from build123d import *

# Parameters (mm, degrees)
BASEHEAD_DEPTH = 13.4
SKETCH4_W      = 0.8
SKETCH4_H      = 12.320508076


# Read off the part's stored shape, not the designer's step: HeadChamfer
with BuildPart() as part:
    # Sketch1 → BaseHead (new body)
    with BuildSketch(Plane(origin=(0, 0, 0), x_dir=(0, 0, -1), z_dir=(1, 0, 0))):
        Polygon((15, 8.660254038), (15, -8.660254038), (0, -17.320508076), (-15, -8.660254038), (-15, 8.660254038), (0, 17.320508076), align=None)
    extrude(amount=BASEHEAD_DEPTH)

    # HeadChamfer outline → HeadChamfer (revolve, cut)
    with BuildSketch(Plane.YX):
        Polygon((17.320508077, 1.339745963), (14.99999979, -1.21e-07), (17.320508077, -1.21e-07), align=None)
    revolve(axis=Axis((0, 0, 0), (1, 0, 0)), mode=Mode.SUBTRACT)

    # HeadChamfer 2 outline → HeadChamfer 2 (revolve)
    with BuildSketch(Plane.YX):
        Polygon((10, 13.4), (10, 172.026), (8.626, 173.4), (0, 173.4), (0, 13.4), align=None)
    revolve(axis=Axis((0, 0, 0), (1, 0, 0)))

    # Sketch4 → BearingFace (revolve, cut)
    with BuildSketch(Plane.XY, mode=Mode.PRIVATE) as bearingface_sk:
        with Locations((13, 21.160254038)):
            Rectangle(SKETCH4_W, SKETCH4_H)
    revolve(bearingface_sk.sketch.rotate(Axis((0, 0, 0), (1, 0, 0)), 90), axis=Axis((0, 0, 0), (1, 0, 0)), mode=Mode.SUBTRACT)


solid = part.part
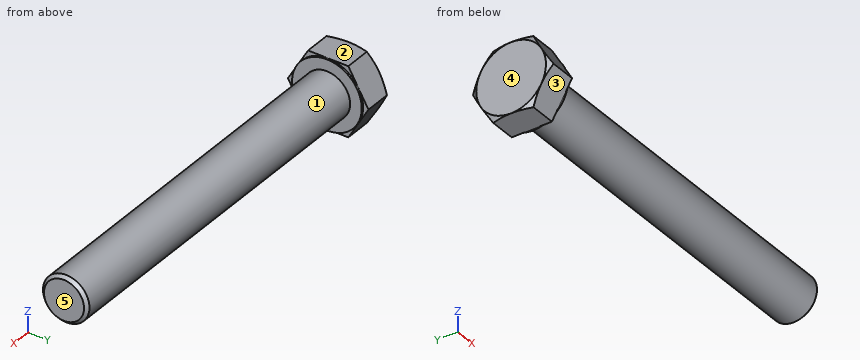
Could you check a few things on this model? Use its own coordinates, in mm. Face numbers are marked on the shaded views. A direction names the side the tool comes from. Give positions to 0.01 mm unless a question says otherwise; leave off trailing zeros. Order: outer loops, then holes, each group sorted by start corner. A loop starts at its lowest first (then second) coordinate and runs counter-clockwise, first axis right, second up. Notation, with made-up numbers: (71, 52) - (78, 52) arc R29 ccw to (78, 77) - close; hole circle Ø10 at (84.25, 26). An arc over 180 degrees is marked (long way). One line per item, written item: value. Start each with the question number.
1. If I drill on probe 1 along X at (y, z) = (10, -5); probe 2 along Z at (x, y) = (89.5, 0); probe 3 along Y at (x, z) = (144.5, 5.5), over which ranges is the centre line in solid material (lowest first)?
2. For the marked faces 1 and 2, which set-ups out of +Z, -Z, +X, -X, +Y, -Y let a thin tool reach every point of the face, with its end or its side?
3. Imagine slicing it at A-A on x = 127. List the corners of the cut face in (y, z) for me, plus the area to 3 significant figures.
4. Thinking about a two-plate mould opening in X: for the marked faces 3, 4 and 5, which applies, +X half, -X half, draft (parallel to the pull), parting line (faces both ways), or undercut?
5. For P1, Ø8, axis at x = 102, y = -2.5, coming from the +Z side; P2, Ø2, axis at y = -4, z = 9.5, coming from the +X side; P3, Ø5, axis at x = 113.5, z = 11, coming from the -Y side, each with a flat end and sliding along its axis, tell me the tip position at first contact or that it passes through.
Values:
1. probe 1: 0 to 13.4
1. probe 2: -10 to 10
1. probe 3: -8.35 to 8.35
2. face 1: +X
2. face 2: +Z, +X, -X, +Y, -Y
3. outline: circle Ø20 at (0, 0)
3. area: 314 mm²
4. face 3: draft
4. face 4: -X half
4. face 5: +X half
5. P1: z = 10
5. P2: x = 172.72
5. P3: y = -5.27
